Could you check a few things on this model? Use its own coordinates, in mm. A direction names the side the tool comes from. Coordinates: 2 decimals unless noted, no trailing zeros. Loops run counter-clockwise (first coordinate to the right, second up) from the corner with the lowest first, then second, coordinate; pieces in that order, holes last. Notation, with made-up numbers: (-37.75, 15) - (-29.75, 15) arc R18 cw to (-29.75, 49) - close; hole circle Ø11 at (-33, 64.5). An arc over 180 degrees is marked (long way). One line per item, written item: value. Start each with the question number.
(1) I'm going to push flat-ended pins straight in: P1, Ø3, axis at x = -2.5, z = 7.5, coming from the +Y side; P2, Ø1.5, axis at x = -5.5, z = 1.5, coming from the -Y side; P3, Ø6, axis at x = 0, z = 8, coming from the -Y side. Where does each tip first touch, or does it pass through?
(2) If I drill on line 1 along X through (y, z) = (-3, 2.5); line 2 along Z through (x, y) = (4.5, 0); line 3 along X through (y, z) = (0, 5.25), over which ranges is the centre line in solid material (lowest first)? Write a range as from..to.
(3) On a 3-axis mill with a long thin cutter (end or side, diameter ignored), from which of +Z, -Z, +X, -X, +Y, -Y can I reach the whole of each face in a straight line? I mean faces 4 (the face through (0, -2.5, 11)), 5 (the face through (0, -2, 6.2)), 6 (the face through (7.18, 1.9, 11.44)), 7 (the face through (-6.449, -1.215, 11.74)). Say none if no direction works.
(4) If we section it at D-D on z = -2.25: Write out the boundary of the cut face in (x, y).
(5) If we section it at A-A on x = -3.25: Write out the boundary of the cut face in (y, z), then the cut area to 3 significant figures.
(6) If we section it at C-C on y = -1.75: Write out the boundary of the cut face in (x, z).
(7) If we mould it in two halves opening along Z, with no side actions, what happens to faces 1 (the face through (-0.11, -1.13, 0.35)), 2 (the face through (6.75, 0, 12)), 3 (the face through (0, -2, 20))? For each: pulls with the +Z half, pulls with the -Z half, needs draft (parallel to the pull), parting line crosses it, or undercut.
(8) If we section it at B-B on y = 1.75: Write out the boundary of the cut face in (x, z), then the cut area to 3 significant figures.
```python
from build123d import *

# Parameters (mm, degrees)
F1_DEPTH = 20
F3_DEPTH = 15.5
F5_W     = 5
F5_H     = 3
F6_DEPTH = 4.5
F7_R     = 1.1815986622
F8_DEPTH = 25


with BuildPart() as f1:
    # F0 (on Top) → F1 (new body)
    with BuildSketch(Plane.XY):
        with BuildLine():
            Line((5.75, 2.5), (-5.75, 2.5))
            ThreePointArc((-5.75, 2.5), (-7.1642135624, 1.9142135624), (-7.75, 0.5))
            Line((-7.75, 0.5), (-7.75, -0.5))
            ThreePointArc((-7.75, -0.5), (-7.1642135624, -1.9142135624), (-5.75, -2.5))
            Line((-5.75, -2.5), (5.75, -2.5))
            ThreePointArc((5.75, -2.5), (7.1642135624, -1.9142135624), (7.75, -0.5))
            Line((7.75, -0.5), (7.75, 0.5))
            ThreePointArc((7.75, 0.5), (7.1642135624, 1.9142135624), (5.75, 2.5))
        make_face()
        with BuildLine():
            ThreePointArc((-6.75, 0.5), (-6.4571067812, 1.2071067812), (-5.75, 1.5))
            Line((-5.75, 1.5), (5.75, 1.5))
            ThreePointArc((5.75, 1.5), (6.4571067812, 1.2071067812), (6.75, 0.5))
            Line((6.75, 0.5), (6.75, -0.5))
            ThreePointArc((6.75, -0.5), (6.4571067812, -1.2071067812), (5.75, -1.5))
            Line((5.75, -1.5), (-5.75, -1.5))
            ThreePointArc((-5.75, -1.5), (-6.4571067812, -1.2071067812), (-6.75, -0.5))
            Line((-6.75, -0.5), (-6.75, 0.5))
        make_face(mode=Mode.SUBTRACT)
    extrude(amount=F1_DEPTH)

    # F2 (on face) → F3 (join)
    with BuildSketch(Plane.YZ.offset(7.75)):
        with BuildLine():
            ThreePointArc((-0.5, 3.9686269666), (-2.6457513111, -3), (4, 0))
            ThreePointArc((4, 0), (3, 2.6457513111), (0.5, 3.9686269666))
            Line((0.5, 3.9686269666), (0.5, 0))
            Line((0.5, 0), (-0.5, 0))
            Line((-0.5, 0), (-0.5, 3.9686269666))
        make_face()
        with BuildLine():
            Line((0.5, 0), (0.5, 3.9686269666))
            ThreePointArc((0.5, 3.9686269666), (0, 4), (-0.5, 3.9686269666))
            Line((-0.5, 3.9686269666), (-0.5, 0))
            Line((-0.5, 0), (0.5, 0))
        make_face()
    extrude(amount=-F3_DEPTH)

    # F5 (on face) → F6 (cut, symmetric)
    with BuildSketch(Plane(origin=(0, 0.6446198131, 0.9206125012), x_dir=(1, 0, 0), z_dir=(0, 0.5735764364, 0.8191520443))):
        with Locations((0, -3.6926725879)):
            Rectangle(F5_W, F5_H)
    extrude(amount=F6_DEPTH, both=True, mode=Mode.SUBTRACT)

    # F7 (on face) → F8 (cut)
    with BuildSketch(Plane(origin=(-7.75, 0, 0), x_dir=(0, -1, 0), z_dir=(-1, 0, 0))):
        Circle(F7_R)
    extrude(amount=-F8_DEPTH, mode=Mode.SUBTRACT)


solid = f1.part
```
Values:
1. P1: stops at y = 2.5
1. P2: stops at y = -3.93
1. P3: stops at y = -2.5
2. line 1: x = -7.75..-2.5, 2.5..7.75
2. line 2: z = -4..-1.18, 1.18..4
2. line 3: x = -7.75..-6.75, 6.75..7.75
3. face 4: +Z, +X, -X, -Y
3. face 5: none
3. face 6: +Z, +X, +Y
3. face 7: +Z
4. outline: (-7.75, -3.31) - (7.75, -3.31) - (7.75, 3.31) - (-7.75, 3.31) - close
5. outline: (-2.5, 3.12) arc R4 ccw (long way) to (2.5, 3.12) - (2.5, 20) - (1.5, 20) - (1.5, 3.71) arc R4 ccw to (-1.5, 3.71) - (-1.5, 20) - (-2.5, 20) - close; hole circle Ø2.36 at (0, 0)
5. area: 79.0 mm2
6. outline: (-7.75, -3.6) - (7.75, -3.6) - (7.75, 3.6) - (7.31, 3.6) - (7.31, 20) - (-7.31, 20) - (-7.31, 3.6) - (-7.75, 3.6) - close; hole (-2.5, 1.32) - (2.5, 1.32) - (2.5, 6.55) - (-2.5, 6.55) - close
7. face 1: undercut
7. face 2: needs draft
7. face 3: pulls with the +Z half
8. outline: (-7.75, -3.6) - (7.75, -3.6) - (7.75, 3.6) - (7.31, 3.6) - (7.31, 20) - (-7.31, 20) - (-7.31, 3.6) - (-7.75, 3.6) - close
8. area: 351 mm2
